Here's the drawing with two shaded views (mm, measured from the low corner). I have some questions. A direction names the side the tool comes from. Coordinates: 2 decimals unless noted, no trailing zeros. Order: outer loops, then holes, each group sorted by start corner. A loop starts at its lowest first (then second) coordinate and runs counter-clockwise, first axis right, second up. Notation, with made-up numbers: (62.5, -32.75) - (77.5, -32.75) arc R25 ccw to (77.5, -11.75) - close; hole circle Ø9 at (86, -24). An arc over 180 degrees is marked (long way). Answer as a JSON object with one key per item and string values. Group by question number.
(1) Imagine slicing it at A-A, the plane y = 5.25. Write out the boundary of the cut face in (x, z).
(2) Which directions (+Z, -Z, +X, -X, +Y, -Y) give clear straight access to the entire face, cutting with the end or side of a thin tool? Please do the marked faces 4, 5 and 6.
(3) We'd pull the mould along X, two halves only. Please class the marked faces 1, 2 and 3: pulls with the +X half, pulls with the -X half, needs draft (parallel to the pull), parting line crosses it, or undercut.
(4) Please list where these lines run through material, in increasing order: probe 1 along Y at (x, z) = (5.25, 8); probe 2 along X at (y, z) = (5, 15); probe 3 along Z at (x, y) = (7.25, 7.5).
(5) Imagine slicing it at C-C, the plane z = 14. Write out the boundary of the cut face in (x, y), and give its area (3 significant figures).
(6) Imagine slicing it at B-B, the plane x = 4. Write out the boundary of the cut face in (y, z).
(7) Will these pins go through, and if not, where does the flat tip stop? P1, Ø3, axis at x = 5.25, y = 5.25, coming from the +Z side; P2, Ø1, axis at y = 5.5, z = 31, coming from the +X side; P3, Ø3, axis at x = 6, y = 6.5, coming from the +Z side; P4, Ø4, axis at x = 5.5, z = 24.5, coming from the +Y side.
(8) Imagine slicing it at D-D, the plane x = 1.5. Write out the boundary of the cut face in (y, z).
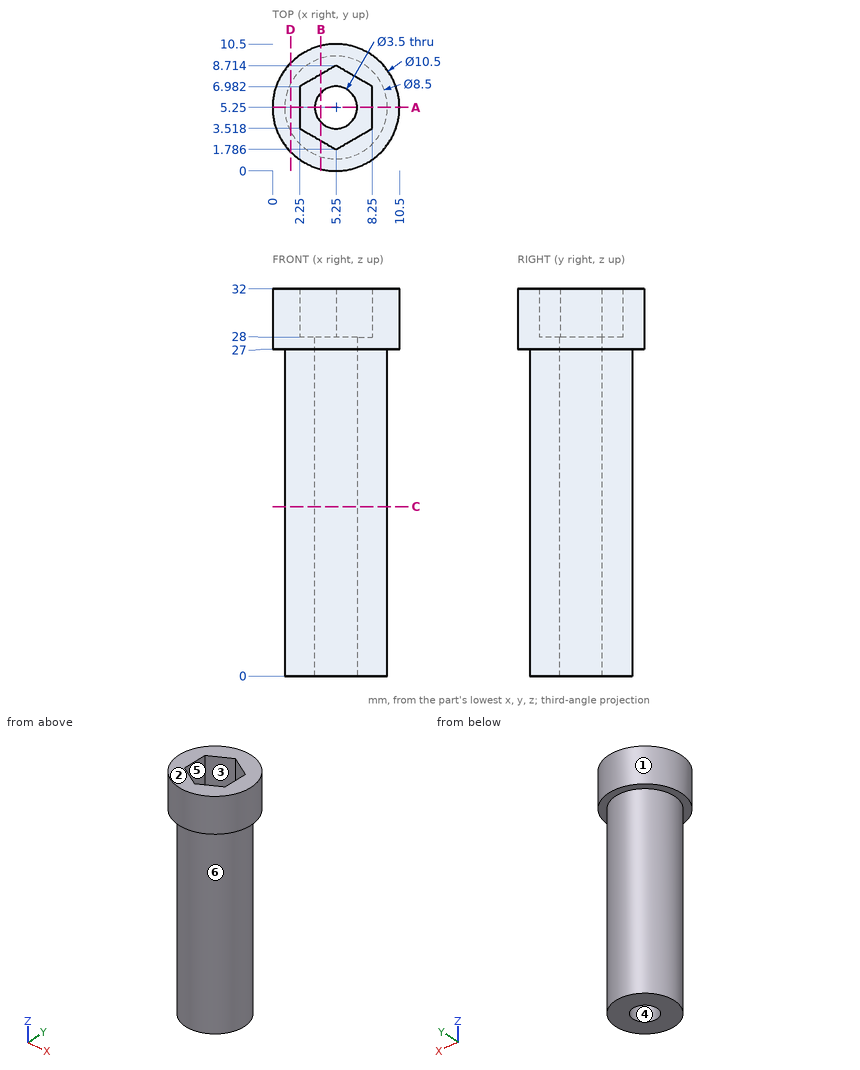
Result set:
{
 "1": {"outline": "(0, 27) - (1, 27) - (1, 0) - (3.5, 0) - (3.5, 28) - (2.25, 28) - (2.25, 32) - (0, 32) - close; (7, 0) - (9.5, 0) - (9.5, 27) - (10.5, 27) - (10.5, 32) - (8.25, 32) - (8.25, 28) - (7, 28) - close"},
 "2": {"face 4": "+Z, -Z", "face 5": "+Z", "face 6": "-Z"},
 "3": {"face 1": "parting line crosses it", "face 2": "needs draft", "face 3": "undercut"},
 "4": {"probe 1": "y = 1 to 3.5, 7 to 9.5", "probe 2": "x = 1.01 to 3.52, 6.98 to 9.49", "probe 3": "z = 0 to 28"},
 "5": {"outline": "circle Ø8.5 at (5.25, 5.25); hole circle Ø3.5 at (5.25, 5.25)", "area": "47.1 mm^2"},
 "6": {"outline": "(0.15, 27) - (1.19, 27) - (1.19, 0) - (4.03, 0) - (4.03, 28) - (2.51, 28) - (2.51, 32) - (0.15, 32) - close; (6.47, 0) - (9.31, 0) - (9.31, 27) - (10.35, 27) - (10.35, 32) - (7.99, 32) - (7.99, 28) - (6.47, 28) - close"},
 "7": {"P1": "passes through", "P2": "stops at x = 10.5", "P3": "stops at z = 28", "P4": "stops at y = 9.5"},
 "8": {"outline": "(1.58, 27) - (3.25, 27) - (3.25, 0) - (7.25, 0) - (7.25, 27) - (8.92, 27) - (8.92, 32) - (1.58, 32) - close"}
}
